Autodesk Inventor part; units mm, degrees
ref_plane "YZ Plane" through (0, 0, 0) normal (1, 0, 0) x (0, 1, 0)
ref_plane "XZ Plane" through (0, 0, 0) normal (0, 1, 0) x (-1, 0, 0)
ref_plane "XY Plane" through (0, 0, 0) normal (0, 0, 1) x (1, 0, 0)
sketch "Sketch1" plane through (0, 0, 0) normal (0, 0, 1) x (1, 0, 0)
  circle A0 centre (0, 0) radius 1.5
  dimension "d0" = 3
extrude "Extrusion1" add sketch "Sketch1" along normal blind 10
sketch "Sketch2" plane through (0, 0, 0) normal (0, 0, -1) x (-1, 0, 0)
  circle A0 centre (0, 0) radius 1.5
  circle A1 centre (0, 0) radius 2.25
  dimension "d3" = 4.5
extrude "Extrusion2" add sketch "Sketch2" along normal blind 3 contours A0 | A1
sketch "Sketch3" plane through (0, 0, -3) normal (0, 0, -1) x (-1, 0, 0)
  circle A0 centre (0, 0) radius 2.25
  line L0 (-0.7217, 1.25) -> (0.7217, 1.25)
  line L1 (0.7217, 1.25) -> (1.4434, 0)
  line L2 (1.4434, 0) -> (0.7217, -1.25)
  line L3 (0.7217, -1.25) -> (-0.7217, -1.25)
  line L4 (-0.7217, -1.25) -> (-1.4434, 0)
  line L5 (-1.4434, 0) -> (-0.7217, 1.25)
  dimension "d6" = 2.5
extrude "Extrusion3" cut sketch "Sketch3" against normal blind 1.5 contours L0 L1 L2 L3 L4 L5
thread "Thread1"
chamfer "Chamfer1" distance 0.508 angle 45 1 edges at (-1.5, 0, 10)
chamfer "Chamfer2" distance 0.25 angle 45 2 edges at (2.25, 0, -3) (2.25, 0, 0)
properties part number "m3 x10" material "Steel"
Part model, mm, in its own coordinate system. A direction names the side the tool comes from. Give positions to 0.01 mm unless a question says otherwise; leave off trailing zeros. Order: outer loops, then holes, each group sorted by start corner. A loop starts at its lowest first (then second) coordinate and runs counter-clockwise, first axis right, second up. Notation, with made-up numbers: (-9, -14.5) - (3, -14.5) arc R23 ccw to (3, 9.5) - close; hole circle Ø5 at (-30.5, 63). An arc over 180 degrees is marked (long way). One line per question, with ' | ' between items.
1. Drill centre lines: probe 1 along Y at (x, z) = (-0.4, 1); probe 2 along Z at (x, y) = (-1.25, 1.2); probe 3 along Z at (x, y) = (0.85, -0.25). Where is each one in solid material? Low to high.
Filled in:
probe 1: -1.45 to 1.45 | probe 2: -3 to 0 | probe 3: -1.5 to 10
2. Which spindle directions (+Z, -Z, +X, -X, +Y, -Y) get a long thin tool onto all of the face, cutting with end or side? Do faces 1 (the face through (-1.088, -0.616, -2.26)), 2 (the face through (-1.5, -0.07, 4.68)). Say none if no direction does.
Filled in:
face 1: -Z | face 2: +Z
3. Band-saw the part on A-A on x = 0. List the corners of the cut face in (y, z), then the cut area to 3 significant figures.
Filled in:
outline: (-2.25, -2.75) - (-2, -3) - (-1.25, -3) - (-1.25, -1.5) - (1.25, -1.5) - (1.25, -3) - (2, -3) - (2.25, -2.75) - (2.25, -0.25) - (2, 0) - (1.5, 0) - (1.5, 9.49) - (0.99, 10) - (-0.99, 10) - (-1.5, 9.49) - (-1.5, 0) - (-2, 0) - (-2.25, -0.25) - close | area: 39.4 mm²
4. Drop flat-ended pins along their axis: P1, Ø1.3, axis at x = -0.5, y = 0, coming from the -Z side; P2, Ø2, axis at x = 0.5, z = 4.5, coming from the +Y side. Give the stop position or say it passes through.
Filled in:
P1: z = -1.5 | P2: y = 1.5
5. Pull direction X, two halves, no side cores. Call faces 3 (the face through (-1.08, 0.63, -2.26)), 4 (the face through (0, 0, 10)), 5 (the face through (0.29, -2.23, -1.48)), 6 (the face through (1.08, -0.63, -2.26)): +X half, -X half, draft (parallel to the pull), parting line (faces both ways), or undercut.
Filled in:
face 3: undercut | face 4: draft | face 5: parting line | face 6: undercut
6. Band-saw the part on B-B on z = 5.25. List the corners of the cut face in (x, y), then the cut area to 3 significant figures.
Filled in:
outline: circle Ø3 at (0, 0) | area: 7.07 mm²
